Read the model definition and answer for the solid it produces. Units are mm, in the model's axes. A direction names the side the tool comes from. Round coordinates to 2 decimals unless told otherwise and drop trailing zeros. Order: outer loops, then holes, each group sorted by start corner. A loop starts at its lowest first (then second) coordinate and runs counter-clockwise, first axis right, second up. Notation, with made-up numbers: (5.25, -34) - (61.25, -34) arc R28 cw to (61.25, -8) - close; hole circle Ø8 at (87.25, -10). An arc over 180 degrees is marked (long way). Answer as a JSON object with one key per item and string values. Group by question number.
Q1. The mould has two halves that part along X. Classify faces 1 (the flat face through (19, -23, 37)), 2 (the flat face through (27, -25, 39.25)), 3 (the flat face through (50.25, -17, 36)), 4 (the flat face through (24.75, -17, 38)): pulls with the +X half, pulls with the -X half, needs draft (parallel to the pull), parting line crosses it, or undercut.
Q2. A cutting plane is placed at C-C on x = 17.5. Determine the outline of the cut face in (y, z), and give its area (3 significant figures).
Q3. A tool of negligible diameter and unlimited length cuts with its end or side. For faces 5 (the flat face through (19, -10.5, 37)), 6 (the flat face through (35, 15, 19)), 7 (the flat face through (35, -32, 36)), from which of +Z, -Z, +X, -X, +Y, -Y can it reach the whole face along a straight path? Write none if from no direction.
Q4. A cutting plane is placed at D-D on z = 22. Determine the outline of the cut face in (x, y).
Q5. A cutting plane is placed at A-A on y = 7.5. Determine the outline of the cut face in (x, z).
Q6. Consider line 1 (Z direction, x = 51.5, y = 0.5); line 2 (Z direction, x = 55.5, y = 6.5); line 3 (Z direction, x = 36, y = -11). Determine where each line is inside the solid, lowest interval first.
Q7. A cutting plane is placed at B-B on x = 5. Determine the outline of the cut face in (y, z), and give its area (3 significant figures).
Q8. Given pin 1 Ø10 at (x, y) = (53, -27.5) entering from -Z; pin 2 Ø2 at (y, z) = (-5, 36.5) entering from +X; pin 3 Ø16.5 at (x, z) = (32, 25) entering from -Y; pin 4 Ø2 at (x, z) = (54.5, 35) entering from -Y, each flat-ended and moving along its own axis, determine where each tip first touches the part or whether it passes through.
```python
from build123d import *

# Parameters (mm, degrees)
SKETCH_W        = 70
SKETCH_H        = 15
SKETCH_R        = 1.6
PAD_DEPTH       = 2
SKETCH001_W     = 40
SKETCH001_H     = 40
PAD001_DEPTH    = 4
SKETCH002_W     = 40
SKETCH002_H     = 49
PAD002_DEPTH    = 5
POCKET_DEPTH    = 2
SKETCH004_W     = 9.75
SKETCH004_H     = 12.5
POCKET001_DEPTH = 1.5
SKETCH005_R     = 0.925
POCKET002_DEPTH = 2.25
FILLET_R        = 1


with BuildPart() as part:
    # Sketch → Pad (new body)
    with BuildSketch(Plane.XY):
        with Locations((35, 7.5)):
            Rectangle(SKETCH_W, SKETCH_H)
        with Locations((5, 3)):
            Circle(SKETCH_R, mode=Mode.SUBTRACT)
        with Locations((65, 3)):
            Circle(SKETCH_R, mode=Mode.SUBTRACT)
    extrude(amount=PAD_DEPTH)

    # Sketch001 (on Face3 of Pad) → Pad001 (join)
    with BuildSketch(Plane(origin=(0, 15, 0), x_dir=(-1, 0, 0), z_dir=(0, 1, 0))):
        with Locations((-35, 20)):
            Rectangle(SKETCH001_W, SKETCH001_H)
    extrude(amount=PAD001_DEPTH)

    # Sketch002 (on Face15 of Pad001) → Pad002 (join)
    with BuildSketch(Plane.XY.offset(40)):
        with Locations((35, -9.5)):
            Rectangle(SKETCH002_W, SKETCH002_H)
    extrude(amount=-PAD002_DEPTH)

    # Sketch003 (on Face15 of Pad002) → Pocket (cut)
    with BuildSketch(Plane(origin=(0, 0, 35), x_dir=(1, 0, 0), z_dir=(0, 0, -1))):
        Polygon((19.75, 32), (50.25, 32), (50.25, 1.5), (19.75, 1.5), (19.75, 10.5), (15, 10.5), (15, 23), (19.75, 23), align=None)
    extrude(amount=-POCKET_DEPTH, mode=Mode.SUBTRACT)

    # Sketch004 (on Face28 of Pocket) → Pocket001 (cut)
    with BuildSketch(Plane(origin=(0, 0, 37), x_dir=(1, 0, 0), z_dir=(0, 0, -1))):
        with Locations((19.875, 16.75)):
            Rectangle(SKETCH004_W, SKETCH004_H)
    extrude(amount=-POCKET001_DEPTH, mode=Mode.SUBTRACT)

    # Sketch005 (on Face31 of Pocket001) → Pocket002 (cut)
    with BuildSketch(Plane(origin=(0, 0, 37), x_dir=(1, 0, 0), z_dir=(0, 0, -1))):
        with Locations((27.25, 24.75)):
            Circle(SKETCH005_R)
        with Locations((42.25, 24.75)):
            Circle(SKETCH005_R)
        with Locations((27.25, 8.75)):
            Circle(SKETCH005_R)
        with Locations((42.25, 8.75)):
            Circle(SKETCH005_R)
    extrude(amount=-POCKET002_DEPTH, mode=Mode.SUBTRACT)

    # Fillet
    fillet_edges = [part.edges().sort_by_distance(p)[0] for p in [
        (70, 0, 1),
        (70, 15, 1),
        (0, 0, 1),
        (0, 15, 1),
        (15, -34, 37.5),
        (55, -34, 37.5),
        (15, 19, 20),
        (55, 19, 20),
    ]]
    fillet(fillet_edges, radius=FILLET_R)


solid = part.part
```
Result set:
{
 "1": {"face 1": "needs draft", "face 2": "undercut", "face 3": "undercut", "face 4": "pulls with the -X half"},
 "2": {"outline": "(-34, 35) - (-23, 35) - (-23, 38.5) - (-10.5, 38.5) - (-10.5, 35) - (15, 35) - (15, 2) - (0, 2) - (0, 0) - (19, 0) - (19, 40) - (-34, 40) - close", "area": "391 mm²"},
 "3": {"face 5": "-Z, -X", "face 6": "+X, -X, -Y", "face 7": "-Z"},
 "4": {"outline": "(15, 15) - (55, 15) - (55, 18) arc R1 ccw to (54, 19) - (16, 19) arc R1 ccw to (15, 18) - close"},
 "5": {"outline": "(0, 0) - (70, 0) - (70, 2) - (0, 2) - close; (15, 35) - (55, 35) - (55, 40) - (15, 40) - close"},
 "6": {"line 1": "z = 0 to 2, 35 to 40", "line 2": "z = 0 to 2", "line 3": "z = 37 to 40"},
 "7": {"outline": "(0, 0) - (1.4, 0) - (1.4, 2) - (0, 2) - close; (4.6, 0) - (15, 0) - (15, 2) - (4.6, 2) - close", "area": "23.6 mm²"},
 "8": {"pin 1": "stops at z = 35", "pin 2": "stops at x = 55", "pin 3": "stops at y = 15", "pin 4": "stops at y = -34"}
}
